Autodesk Inventor part; units mm, degrees
ref_plane "YZ Plane" through (0, 0, 0) normal (1, 0, 0) x (0, 1, 0)
ref_plane "XZ Plane" through (0, 0, 0) normal (0, 1, 0) x (-1, 0, 0)
ref_plane "XY Plane" through (0, 0, 0) normal (0, 0, 1) x (1, 0, 0)
sketch "Sketch1" plane through (0, 0, 0) normal (0, 0, 1) x (1, 0, 0)
  arc A0 (-88.3243, -23.6664) -> (88.3243, -23.6664) centre (0, 0) ccw
  line L0 (-25.4, 76.2) -> (25.4, 76.2)
  line L1 (25.4, 76.2) -> (25.4, -6.8059)
  line L2 (-25.4, -6.8059) -> (-25.4, 76.2)
  line L3 (-25.4, -6.8059) -> (-88.3243, -23.6664)
  line L4 (25.4, -6.8059) -> (88.3243, -23.6664)
  line L5 (0, -124.968) -> (0, 109.728)
extrude "Extrusion1" add sketch "Sketch1" against normal mid plane 25.4
sketch "Sketch2" plane through (0, 0, -12.7) normal (0, 0, -1) x (-1, 0, 0)
  circle A0 centre (0, 0) radius 15.24
  circle A1 centre (0, 0) radius 20.32
  dimension "d7" = 30.48
  dimension "d8" = 40.64
extrude "Extrusion2" cut sketch "Sketch2" against normal through all contours A0
extrude "Extrusion3" add sketch "Sketch2" along normal blind 2.54 contours A0 | A1
sketch "Sketch3" plane through (0, 0, 12.7) normal (0, 0, 1) x (1, 0, 0)
  circle A0 centre (0, 45.72) radius 15.24
  circle A1 centre (0, 45.72) radius 20.32
  point P0 (0, 0)
  dimension "d13" = 30.48
  dimension "d14" = 40.64
  dimension "d15" = 45.72
extrude "Extrusion4" cut sketch "Sketch3" against normal through all contours A0
extrude "Extrusion5" add sketch "Sketch3" along normal blind 2.54 contours A0 | A1
sketch "Sketch4" plane through (0, 0, 12.7) normal (0, 0, 1) x (1, 0, 0)
  arc A0 (-73.3333, -40.5957) -> (73.3333, -40.5957) centre (0, 0) ccw
  circle A1 centre (0, 45.72) radius 20.32
  circle A2 centre (0, 45.72) radius 15.24
  circle A3 centre (0, 0) radius 15.24
  line L0 (25.4, -6.8059) -> (88.3243, -23.6664)
  arc A4 (-88.3243, -23.6664) -> (88.3243, -23.6664) centre (0, 0) ccw
  line L1 (-88.3243, -23.6664) -> (-25.4, -6.8059)
  line L2 (-25.4, -6.8059) -> (-25.4, 76.2)
  line L3 (-25.4, 76.2) -> (25.4, 76.2)
  line L4 (25.4, 76.2) -> (25.4, -6.8059)
  circle A5 centre (0, 45.72) radius 20.32
  circle A6 centre (0, 0) radius 15.24
  arc A7 (-88.3243, -23.6664) -> (88.3243, -23.6664) centre (0, 0) ccw
  line L5 (88.3243, -23.6664) -> (25.4, -6.8059)
  line L6 (25.4, -6.8059) -> (25.4, 76.2)
  line L7 (25.4, 76.2) -> (-25.4, 76.2)
  line L8 (-25.4, 76.2) -> (-25.4, -6.8059)
  line L9 (-25.4, -6.8059) -> (-88.3243, -23.6664)
  line L10 (-67.074, -25.8612) -> (-23.4361, -14.1685)
  line L11 (23.4361, -14.1685) -> (67.074, -25.8612)
  arc A8 (-67.074, -25.8612) -> (-73.3333, -40.5957) centre (-64.4444, -35.675) ccw
  arc A9 (73.3333, -40.5957) -> (67.074, -25.8612) centre (64.4444, -35.675) ccw
  arc A10 (-14.1484, -16.308) -> (14.1484, -16.308) centre (0, 0) ccw
  arc A11 (-14.1484, -16.308) -> (-23.4361, -14.1685) centre (-20.8065, -23.9823) ccw
  arc A12 (23.4361, -14.1685) -> (14.1484, -16.308) centre (20.8065, -23.9823) ccw
  point P0 (78.6564, -28.9647)
  point P1 (-78.6564, -28.9647)
  point P2 (-17.5401, -12.5887)
  point P3 (17.5401, -12.5887)
  dimension "d20" = 167.64
  dimension "d21" = 7.62
  dimension "d22" = 7.62
  dimension "d23" = 10.16
  dimension "d24" = 43.18
  dimension "d25" = 10.16
extrude "Extrusion6" cut sketch "Sketch4" against normal blind 5.08 contours A8 L10 A11 A10 A12 L11 A9 A0
mirror "Mirror1" about plane through (0, 0, 0) normal (0, 0, 1) of "Extrusion6"
sketch "Sketch5" plane through (0, 0, 0) normal (1, 0, 0) x (0, 1, 0)
  line L0 (-20.32, -15.24) -> (-20.32, -12.7)
  line L1 (-20.32, -12.7) -> (-21.59, -12.7)
  line L2 (-21.59, -12.7) -> (-21.59, -7.62)
  line L3 (-21.59, -7.62) -> (-83.82, -7.62)
  line L4 (-83.82, -7.62) -> (-83.82, -12.7)
  line L5 (-83.82, -12.7) -> (-91.44, -12.7)
  line L6 (-91.44, -12.7) -> (-91.44, 12.7)
  line L7 (-91.44, 12.7) -> (-83.82, 12.7)
  line L8 (-83.82, 12.7) -> (-83.82, 7.62)
  line L9 (-83.82, 7.62) -> (-21.59, 7.62)
  line L10 (-21.59, 7.62) -> (-21.59, 12.7)
  line L11 (-21.59, 12.7) -> (-15.24, 12.7)
  line L12 (-15.24, 12.7) -> (-15.24, -12.7)
  line L13 (-15.24, -12.7) -> (15.24, -12.7)
  line L14 (15.24, -12.7) -> (15.24, 12.7)
  line L15 (15.24, 12.7) -> (25.4, 12.7)
  line L16 (25.4, 12.7) -> (25.4, 15.24)
  line L17 (25.4, 15.24) -> (66.04, 15.24)
  line L18 (66.04, 15.24) -> (66.04, 12.7)
  line L19 (66.04, 12.7) -> (76.2, 12.7)
  line L20 (76.2, 12.7) -> (76.2, -12.7)
  line L21 (76.2, -12.7) -> (60.96, -12.7)
  line L22 (60.96, -12.7) -> (60.96, 12.7)
  line L23 (60.96, 12.7) -> (30.48, 12.7)
  line L24 (30.48, 12.7) -> (30.48, -12.7)
  line L25 (30.48, -12.7) -> (20.32, -12.7)
  line L26 (20.32, -12.7) -> (20.32, -15.24)
  line L27 (20.32, -15.24) -> (-20.32, -15.24)
  line L28 (76.2, -12.7) -> (76.2, 12.7)
  line L29 (-6.8059, -12.7) -> (76.2, -12.7)
  line L30 (-6.8059, -12.7) -> (-6.8059, 12.7)
  line L31 (76.2, 12.7) -> (-6.8059, 12.7)
  line L32 (-23.6664, 12.7) -> (-23.6664, -12.7)
  line L33 (-23.6664, -12.7) -> (-23.6664, -12.7)
  line L34 (-23.6664, -12.7) -> (-23.6664, 12.7)
  line L35 (-23.6664, 12.7) -> (-23.6664, 12.7)
  circle A0 centre (45.72, 0) radius 3.81
  circle A1 centre (0, 0) radius 3.81
  dimension "d28" = 7.62
  dimension "d29" = 7.62
extrude "Extrusion7" cut sketch "Sketch5" against normal through all both and the other way through all contours A0 | A1
fillet "Fillet1" radius 2.54 16 edges at (-73.7957, -31.7026, 7.62) (-45.2551, -20.0149, 7.62) (-18.5258, -14.0816, 7.62) (0, -21.59, 7.62) (18.5258, -14.0816, 7.62) (45.2551, -20.0149, 7.62) (73.7957, -31.7026, 7.62) (0, -83.82, 7.62) (-73.7957, -31.7026, -7.62) (-45.2551, -20.0149, -7.62) (-18.5258, -14.0816, -7.62) (0, -21.59, -7.62) (18.5258, -14.0816, -7.62) (45.2551, -20.0149, -7.62) (73.7957, -31.7026, -7.62) (0, -83.82, -7.62)
equation "\"BendRadius\" = Thickness"
equation "\"BendReliefWidth\" = Thickness"
equation "\"BendReliefDepth\" = 0.5 * Thickness"
equation "\"CornerReliefSize\" = 4 * Thickness"
equation "\"MinimumRemnant\" = 2 * Thickness"
equation "\"TransitionRadius\" = BendRadius"
equation "\"JacobiRadiusSize\" = BendRadius"
equation "\"GapSize\" = Thickness"
properties part number "crankshaft counterwieght"
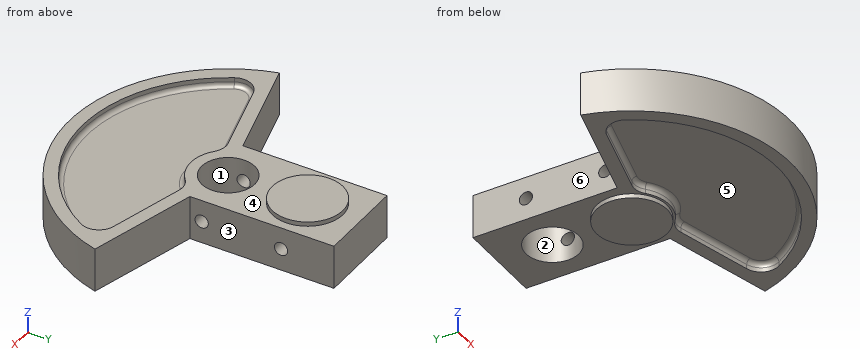
For this review, take the finished solid that the model builds, in its own axes (mm). Face numbers are marked on the shaded views. A direction names the side the tool comes from. Coordinates: 2 decimals unless noted, no trailing zeros. Order: outer loops, then holes, each group sorted by start corner. A loop starts at its lowest first (then second) coordinate and runs counter-clockwise, first axis right, second up. Notation, with made-up numbers: (89, -33) - (112, -33) arc R19 cw to (112, -14) - close; hole circle Ø9 at (84.25, -38). An arc over 180 degrees is marked (long way). Answer as CSV lines item,"result". Start each with the question number.
1) Draft analysis for pull direction X (two halves, no side actions). For the marked faces 4, 5 and 6, state which applies: +X half, -X half, draft (parallel to the pull), parting line (faces both ways), or undercut.
2) Add section A-A (z = 0). State the section outline as (x, y) points, then the cut area to 3 significant figures.
3) To check wall thickness, follow line 1 along Y through (x, z) = (0, 3); line 2 along Z through (x, y) = (-22, 45.72); line 3 along Y through (x, z) = (21, 0). State the ranges of each line that lie inside material, in increasing order. Write a range as [from, to].
4) Machinability: for the marked faces 1, 2 and 3, which of the approach directions +Z, -Z, +X, -X, +Y, -Y give a long, thin tool a straight path to every point of the face, cutting with its end or side? Answer none if there is none.
5) Add section B-B (y = 0). State the section outline as (x, z) points, then the cut area to 3 significant figures.
6) Insertion check: P1, Ø7, axis at y = 45.72, z = 0, coming from the +X side; P2, Ø7.5, axis at y = 27.5, z = -3, coming from the -X side; P3, Ø2, axis at x = 69.5, z = -11.5, coming from the +Y side; P4, Ø12, axis at y = 0, z = 0, coming from the +X side. Each pin has a flat end and moves straight along its axis. Give the tip position at first contact, or say it passes through.
7) Add section D-D (y = 36). State the section outline as (x, z) points.
Result:
1,face 4,"draft"
1,face 5,"undercut"
1,face 6,"-X half"
2,outline,"(-88.32, -23.67) arc R91.44 ccw to (88.32, -23.67) - (25.4, -6.81) - (25.4, -3.81) - (14.76, -3.81) arc R15.24 cw to (-14.76, -3.81) - (-25.4, -3.81) - (-25.4, -6.81) - close; (-25.4, 3.81) - (-14.76, 3.81) arc R15.24 cw to (14.76, 3.81) - (25.4, 3.81) - (25.4, 41.91) - (14.76, 41.91) arc R15.24 cw to (-14.76, 41.91) - (-25.4, 41.91) - close; (-25.4, 49.53) - (-14.76, 49.53) arc R15.24 cw to (14.76, 49.53) - (25.4, 49.53) - (25.4, 76.2) - (-25.4, 76.2) - close"
2,area,"13,200 mm^2"
3,line 1,"[-91.44, -15.24], [15.24, 30.48], [60.96, 76.2]"
3,line 2,"[-12.7, -3.81], [3.81, 12.7]"
3,line 3,"[-89, -3.81], [3.81, 41.91], [49.53, 76.2]"
4,face 1,"+Z"
4,face 2,"-Z"
4,face 3,"+Z, -Z, +X, +Y"
5,outline,"(-25.4, -12.7) - (-20.32, -12.7) - (-20.32, -15.24) - (20.32, -15.24) - (20.32, -12.7) - (25.4, -12.7) - (25.4, -3.81) - (15.24, -3.81) - (15.24, -12.7) - (-15.24, -12.7) - (-15.24, -3.81) - (-25.4, -3.81) - close; (-25.4, 3.81) - (-15.24, 3.81) - (-15.24, 12.7) - (-25.4, 12.7) - close; (15.24, 3.81) - (25.4, 3.81) - (25.4, 12.7) - (15.24, 12.7) - close"
5,area,"465 mm^2"
6,P1,"through"
6,P2,"x = -25.4"
6,P3,"y = -18.35"
6,P4,"x = 25.4"
7,outline,"(-25.4, -12.7) - (-11.74, -12.7) - (-11.74, 12.7) - (11.74, 12.7) - (11.74, -12.7) - (25.4, -12.7) - (25.4, 12.7) - (17.84, 12.7) - (17.84, 15.24) - (-17.84, 15.24) - (-17.84, 12.7) - (-25.4, 12.7) - close"
